from build123d import *

# Parameters (mm, degrees)
SKETCH1_W           = 42
SKETCH1_H           = 42
BOSS_EXTRUDE1_DEPTH = 11
CHAMFER1_SIZE       = 4.5
CUT_EXTRUDE1_REACH  = 33.67
SKETCH3_R           = 1.5
CUT_EXTRUDE2_REACH  = 33.67
SKETCH4_R           = 11.2


with BuildPart() as part:
    # Sketch1 → Boss-Extrude1 (new body)
    with BuildSketch(Plane(origin=(0, 0, 0), x_dir=(1, 0, 0), z_dir=(0, 1, 0))):
        Rectangle(SKETCH1_W, SKETCH1_H)
    extrude(amount=BOSS_EXTRUDE1_DEPTH)

    # Chamfer1
    chamfer1_edges = [part.edges().sort_by_distance(p)[0] for p in [
        (21, 5.5, 21),
        (-21, 5.5, 21),
        (-21, 5.5, -21),
        (21, 5.5, -21),
    ]]
    chamfer(chamfer1_edges, length=CHAMFER1_SIZE)

    # Sketch3 → Cut-Extrude1 (cut, up to next)
    with BuildSketch(Plane(origin=(0, 11, 0), x_dir=(1, 0, 0), z_dir=(0, 1, 0)), mode=Mode.PRIVATE) as cut_extrude1_sk1:
        with Locations(Location((-15.5, 15.5, 0), (0, 0, 270))):
            Circle(SKETCH3_R)
    cut_extrude1_tool1 = extrude(cut_extrude1_sk1.sketch, amount=-CUT_EXTRUDE1_REACH, mode=Mode.PRIVATE) & part.part
    # Sketch3 → Cut-Extrude1 (cut, up to next)
    with BuildSketch(Plane(origin=(0, 11, 0), x_dir=(1, 0, 0), z_dir=(0, 1, 0)), mode=Mode.PRIVATE) as cut_extrude1_sk2:
        with Locations(Location((15.5, 15.5, 0), (0, 0, 270))):
            Circle(SKETCH3_R)
    cut_extrude1_tool2 = extrude(cut_extrude1_sk2.sketch, amount=-CUT_EXTRUDE1_REACH, mode=Mode.PRIVATE) & part.part
    # Sketch3 → Cut-Extrude1 (cut, up to next)
    with BuildSketch(Plane(origin=(0, 11, 0), x_dir=(1, 0, 0), z_dir=(0, 1, 0)), mode=Mode.PRIVATE) as cut_extrude1_sk3:
        with Locations(Location((15.5, -15.5, 0), (0, 0, 270))):
            Circle(SKETCH3_R)
    cut_extrude1_tool3 = extrude(cut_extrude1_sk3.sketch, amount=-CUT_EXTRUDE1_REACH, mode=Mode.PRIVATE) & part.part
    # Sketch3 → Cut-Extrude1 (cut, up to next)
    with BuildSketch(Plane(origin=(0, 11, 0), x_dir=(1, 0, 0), z_dir=(0, 1, 0)), mode=Mode.PRIVATE) as cut_extrude1_sk4:
        with Locations(Location((-15.5, -15.5, 0), (0, 0, 270))):
            Circle(SKETCH3_R)
    cut_extrude1_tool4 = extrude(cut_extrude1_sk4.sketch, amount=-CUT_EXTRUDE1_REACH, mode=Mode.PRIVATE) & part.part
    add(cut_extrude1_tool1.solids().sort_by_distance((-15.5, 11, -15.5))[0], mode=Mode.SUBTRACT)
    add(cut_extrude1_tool2.solids().sort_by_distance((15.5, 11, -15.5))[0], mode=Mode.SUBTRACT)
    add(cut_extrude1_tool3.solids().sort_by_distance((15.5, 11, 15.5))[0], mode=Mode.SUBTRACT)
    add(cut_extrude1_tool4.solids().sort_by_distance((-15.5, 11, 15.5))[0], mode=Mode.SUBTRACT)

    # Sketch4 → Cut-Extrude2 (cut, up to next)
    with BuildSketch(Plane(origin=(0, 11, 0), x_dir=(1, 0, 0), z_dir=(0, 1, 0)), mode=Mode.PRIVATE) as cut_extrude2_sk1:
        with Locations(Location((0, 0, 0), (0, 0, 270))):
            Circle(SKETCH4_R)
    cut_extrude2_tool1 = extrude(cut_extrude2_sk1.sketch, amount=-CUT_EXTRUDE2_REACH, mode=Mode.PRIVATE) & part.part
    add(cut_extrude2_tool1.solids().sort_by_distance((0, 11, 0))[0], mode=Mode.SUBTRACT)


solid = part.part
The model under review builds one solid part; all positions refer to its coordinate system, in mm. Give positions to 0.01 mm unless a question says otherwise; leave off trailing zeros. Loops run counter-clockwise (first coordinate to the right, second up) from the corner with the lowest first, then second, coordinate; pieces in that order, holes last. Notation, with made-up numbers: (66, 11) -> (108, 11) arc R27 cw to (108, 36) -> close; hole circle Ø3 at (-32, -36). An arc over 180 degrees is marked (long way). Answer as a JSON object with one key per item and string values. Group by question number.
Q1. Draft analysis for pull direction X (two halves, no side actions). For faces 1 (the flat face through (18.8, 5.4, 18.7)), 2 (the cylindrical face through (15.57, 5.58, 14)), 3 (the flat face through (-18.7, 5.4, 18.8)), state which applies: pulls with the +X half, pulls with the -X half, needs draft (parallel to the pull), parting line crosses it, or undercut.
Q2. Take a section at B-B (y = 7.75). Write out the cut boundary in (x, z), plus the area to 3 significant figures.
Q3. Take a section at A-A (z = 0). Write out the cut boundary in (x, y), plus the area to 3 significant figures.
Q4. Take a section at C-C (x = 0). Write out the cut boundary in (y, z).
Q5. Wall thickness on line 1 along X through (y, z) = (7, -15.5); line 2 along X through (y, z) = (5, 16.5); line 3 along X through (y, z) = (3, 0): over which ranges is each line inside the solid? List them lowest first.
Q6. Insertion check: pin 1 (1.8 mm diameter, centred on x = -15.5, z = 15.5, fed in from +Y); pin 2 (3.5 mm diameter, centred on x = -15.5, z = -15.5, fed in from -Y). Each pin has a flat end and moves straight along its axis. Give the tip position at first contact, or say it passes through.
Q7. Take a section at D-D (x = -15.5). Write out the cut boundary in (y, z).
Answer below:
{
 "1": {"face 1": "pulls with the +X half", "face 2": "undercut", "face 3": "pulls with the -X half"},
 "2": {"outline": "(-21, -16.5) -> (-16.5, -21) -> (16.5, -21) -> (21, -16.5) -> (21, 16.5) -> (16.5, 21) -> (-16.5, 21) -> (-21, 16.5) -> close; hole circle Ø3 at (-15.5, -15.5); hole circle Ø3 at (-15.5, 15.5); hole circle Ø22.4 at (0, 0); hole circle Ø3 at (15.5, -15.5); hole circle Ø3 at (15.5, 15.5)", "area": "1,300 mm2"},
 "3": {"outline": "(-21, 0) -> (-11.2, 0) -> (-11.2, 11) -> (-21, 11) -> close; (11.2, 0) -> (21, 0) -> (21, 11) -> (11.2, 11) -> close", "area": "216 mm2"},
 "4": {"outline": "(0, -21) -> (11, -21) -> (11, -11.2) -> (0, -11.2) -> close; (0, 11.2) -> (11, 11.2) -> (11, 21) -> (0, 21) -> close"},
 "5": {"line 1": "x = -21 to -17, -14 to 14, 17 to 21", "line 2": "x = -21 to -16.62, -14.38 to 14.38, 16.62 to 21", "line 3": "x = -21 to -11.2, 11.2 to 21"},
 "6": {"pin 1": "passes through", "pin 2": "stops at y = 0"},
 "7": {"outline": "(0, -21) -> (11, -21) -> (11, -17) -> (0, -17) -> close; (0, -14) -> (11, -14) -> (11, 14) -> (0, 14) -> close; (0, 17) -> (11, 17) -> (11, 21) -> (0, 21) -> close"}
}
